from build123d import *

# Parameters (mm, degrees)
SKETCH1_R           = 3.25
SKETCH1_R_2         = 2.4
BOSS_EXTRUDE1_DEPTH = 2.2
SKETCH2_R           = 3.9
BOSS_EXTRUDE2_DEPTH = 1
BOSS_EXTRUDE3_START = 1.6
SKETCH3_R           = 2.4
SKETCH3_R_2         = 1.6
BOSS_EXTRUDE3_DEPTH = 1.6
SKETCH4_R           = 1.6
CUT_EXTRUDE1_DEPTH  = 7.376519427


with BuildPart() as part:
    # Sketch1 → Boss-Extrude1 (new body)
    with BuildSketch(Plane(origin=(0, 0, 0), x_dir=(1, 0, 0), z_dir=(0, 1, 0))):
        with Locations(Location((0, 0, 0), (0, 0, 270))):
            Circle(SKETCH1_R)
        with Locations(Location((0, 0, 0), (0, 0, 270))):
            Circle(SKETCH1_R_2, mode=Mode.SUBTRACT)
    extrude(amount=BOSS_EXTRUDE1_DEPTH)

    # Sketch2 → Boss-Extrude2 (add)
    with BuildSketch(Plane.XZ):
        with Locations(Location((0, 0, 0), (0, 0, 270))):
            Circle(SKETCH2_R)
    extrude(amount=BOSS_EXTRUDE2_DEPTH)

    # Sketch3 → Boss-Extrude3 (add)
    with BuildSketch(Plane.XZ.offset(1).offset(BOSS_EXTRUDE3_START)):
        with Locations(Location((0, 0, 0), (0, 0, 90))):
            Circle(SKETCH3_R)
        with Locations(Location((0, 0, 0), (0, 0, 270))):
            Circle(SKETCH3_R_2, mode=Mode.SUBTRACT)
    extrude(amount=-BOSS_EXTRUDE3_DEPTH)

    # Sketch4 → Cut-Extrude1 (cut, through all)
    with BuildSketch(Plane.XZ.offset(1)):
        with Locations(Location((0, 0, 0), (0, 0, 270))):
            Circle(SKETCH4_R)
    extrude(amount=-CUT_EXTRUDE1_DEPTH, mode=Mode.SUBTRACT)


solid = part.part
The listing builds one solid part. Answer for the finished solid, in the listing's coordinates (mm). A direction names the side the tool comes from. Give positions to 0.01 mm unless a question says otherwise; leave off trailing zeros. Write each loop counter-clockwise with the first axis right and the second up, starting at its lowest first coordinate (ties: lowest second). Pieces come first, ordered by that corner, then holes.
Item 1: Section B-B, the plane x = 0 is taken. Write down the section's boundary in (y, z), plus the area to 3 significant figures.
Item 2: Section A-A, the plane z = 0 is taken. Write down the section's boundary in (x, y), plus the area to 3 significant figures.
Item 3: Determine the mould class of faces 1 (the cylindrical face through (-0.97, -1.32, 1.27)), 2 (the cylindrical face through (-1.978, 1.085, -2.579)), 3 (the flat face through (3, 0, 2)) for opening direction X: released by +X, released by -X, zero draft, split by the parting line, or undercut.
Item 4: Section D-D, the plane x = 2.25 is taken. Write down the section's boundary in (y, z).
Item 5: Which of the six approach directions +Z, -Z, +X, -X, +Y, -Y give full straight-line access (tool end or side, diameter ignored) to faces 4 (the flat face through (2, -2.6, 0)), 5 (the cylindrical face through (-2.024, -1.811, 1.29)), 6 (the flat face through (-2, 0, 0))?
Item 6: Section C-C, the plane y = -0.4 is taken. Write down the section's boundary in (x, z), plus the area to 3 significant figures.
Item 7: Flat-ended cylindrical pins translate along their axes: P1, Ø2.5, axis at x = 0.5, z = -0.5, coming from the +Y side; P2, Ø1, axis at x = -1, z = 3, coming from the -Y side. Find the tip coordinate at first contact, or state that the pin passes through.
Item 8: Find the intervals of material crossed by line 1 along X through (y, z) = (-0.7, 0); line 2 along X through (y, z) = (-1.3, 0); line 3 along Y through (x, z) = (-2.75, 2.5), in increasing order.
Completed:
1. outline: (-2.6, -2.4) - (-1, -2.4) - (-1, -3.9) - (0, -3.9) - (0, -3.25) - (2.2, -3.25) - (2.2, -2.4) - (0, -2.4) - (0, -1.6) - (-2.6, -1.6) - close; (-2.6, 1.6) - (0, 1.6) - (0, 2.4) - (2.2, 2.4) - (2.2, 3.25) - (0, 3.25) - (0, 3.9) - (-1, 3.9) - (-1, 2.4) - (-2.6, 2.4) - close
1. area: 10.9 mm2
2. outline: (-3.9, -1) - (-2.4, -1) - (-2.4, -2.6) - (-1.6, -2.6) - (-1.6, 0) - (-2.4, 0) - (-2.4, 2.2) - (-3.25, 2.2) - (-3.25, 0) - (-3.9, 0) - close; (1.6, -2.6) - (2.4, -2.6) - (2.4, -1) - (3.9, -1) - (3.9, 0) - (3.25, 0) - (3.25, 2.2) - (2.4, 2.2) - (2.4, 0) - (1.6, 0) - close
2. area: 10.9 mm2
3. face 1: undercut
3. face 2: split by the parting line
3. face 3: zero draft
4. outline: (-2.6, -0.84) - (-1, -0.84) - (-1, -3.19) - (0, -3.19) - (0, -2.35) - (2.2, -2.35) - (2.2, -0.84) - (0, -0.84) - (0, 0.84) - (2.2, 0.84) - (2.2, 2.35) - (0, 2.35) - (0, 3.19) - (-1, 3.19) - (-1, 0.84) - (-2.6, 0.84) - close
5. face 4: +Z, -Z, +X, -X, -Y
5. face 5: -Y
5. face 6: +Y
6. outline: circle Ø7.8 at (0, 0); hole circle Ø3.2 at (0, 0)
6. area: 39.7 mm2
7. P1: stops at y = 0
7. P2: stops at y = -1
8. line 1: x = -3.9 to -1.6, 1.6 to 3.9
8. line 2: x = -2.4 to -1.6, 1.6 to 2.4
8. line 3: y = -1 to 0
